The figure shows three views and two pictorial views of one solid part (mm, origin at its lowest corner). Answer the questions. Give positions to 0.01 mm unless a question says otherwise; leave off trailing zeros. Order: outer loops, then holes, each group sorted by start corner. A loop starts at its lowest first (then second) coordinate and runs counter-clockwise, first axis right, second up. Notation, with made-up numbers: (44, 24) - (87, 24) arc R23 cw to (87, 38) - close; hole circle Ø6 at (-4, -33.5). An arc over 180 degrees is marked (long way). Use a Markdown table: item, result. Add a question column.
1. Flat-ended cylindrical pins translate along their axes: P1, Ø1, axis at x = 1, z = 1, coming from the -Y side (3 decimals); P2, Ø1.6, axis at y = 2, z = 2, coming from the -X side (3 decimals); P3, Ø1.5, axis at y = 34, z = 0.5, coming from the +X side. Find the tip coordinate at first contact, or state that the pin passes through.
2. A cutting plane is placed at A-A on z = 1.4. Determine the outline of the cut face in (x, y) (3 decimals), and give its area (3 significant figures).
3. A cutting plane is placed at C-C on x = 26. Determine the outline of the cut face in (y, z) (3 decimals).
4. Consider L1, parallel to X at y = 8, z = 0.65; L2, parallel to Y at x = 51, z = 1.2 (1 decimal); L3, parallel to Y at x = 13.5, z = 1.85 (3 decimals). Determine where each line is inside the solid, lowest interval first.
5. A cutting plane is placed at B-B on y = 29.5. Determine the outline of the cut face in (x, z) (3 decimals), and give its area (3 significant figures).
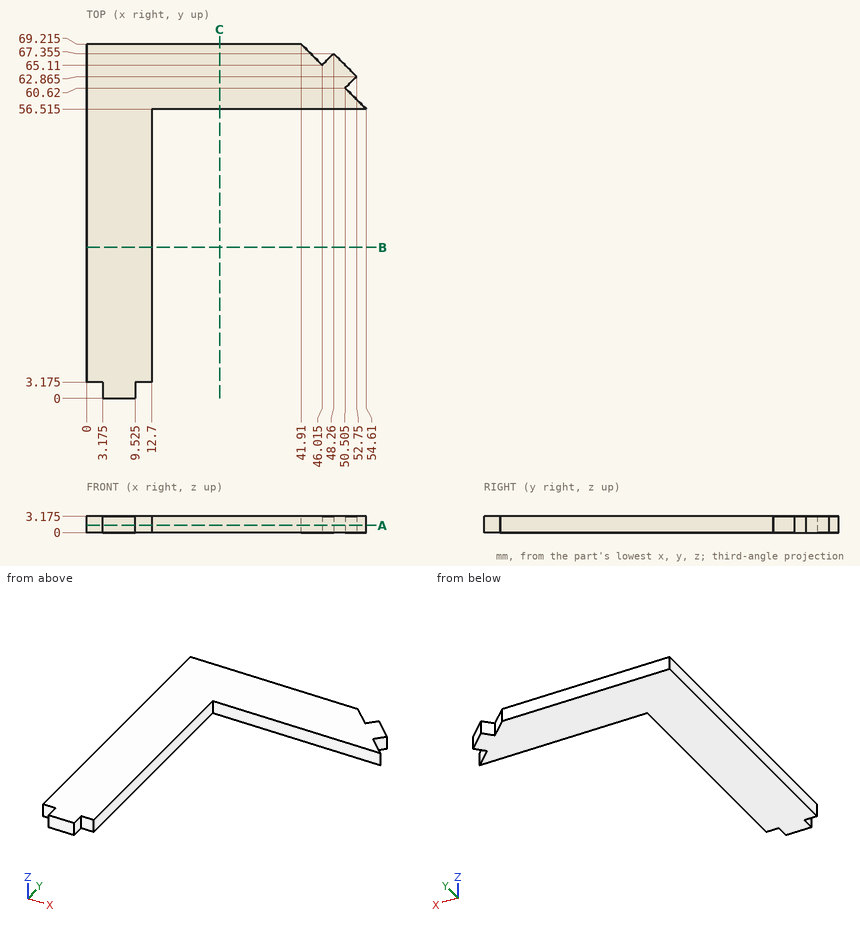
Output values:
| question | item | result |
|---|---|---|
| 1 | P1 | y = 3.175 |
| 1 | P2 | x = 3.175 |
| 1 | P3 | x = 12.7 |
| 2 | outline | (0, 3.175) - (3.175, 3.175) - (3.175, 0) - (9.525, 0) - (9.525, 3.175) - (12.7, 3.175) - (12.7, 56.515) - (54.61, 56.515) - (50.505, 60.62) - (52.75, 62.865) - (48.26, 67.355) - (46.015, 65.11) - (41.91, 69.215) - (0, 69.215) - close |
| 2 | area | 1,330 mm² |
| 3 | outline | (56.515, 0) - (69.215, 0) - (69.215, 3.175) - (56.515, 3.175) - close |
| 4 | L1 | 0 to 12.7 |
| 4 | L2 | 56.5 to 60.1, 61.1 to 64.6 |
| 4 | L3 | 56.515 to 69.215 |
| 5 | outline | (0, 0) - (12.7, 0) - (12.7, 3.175) - (0, 3.175) - close |
| 5 | area | 40.3 mm² |
